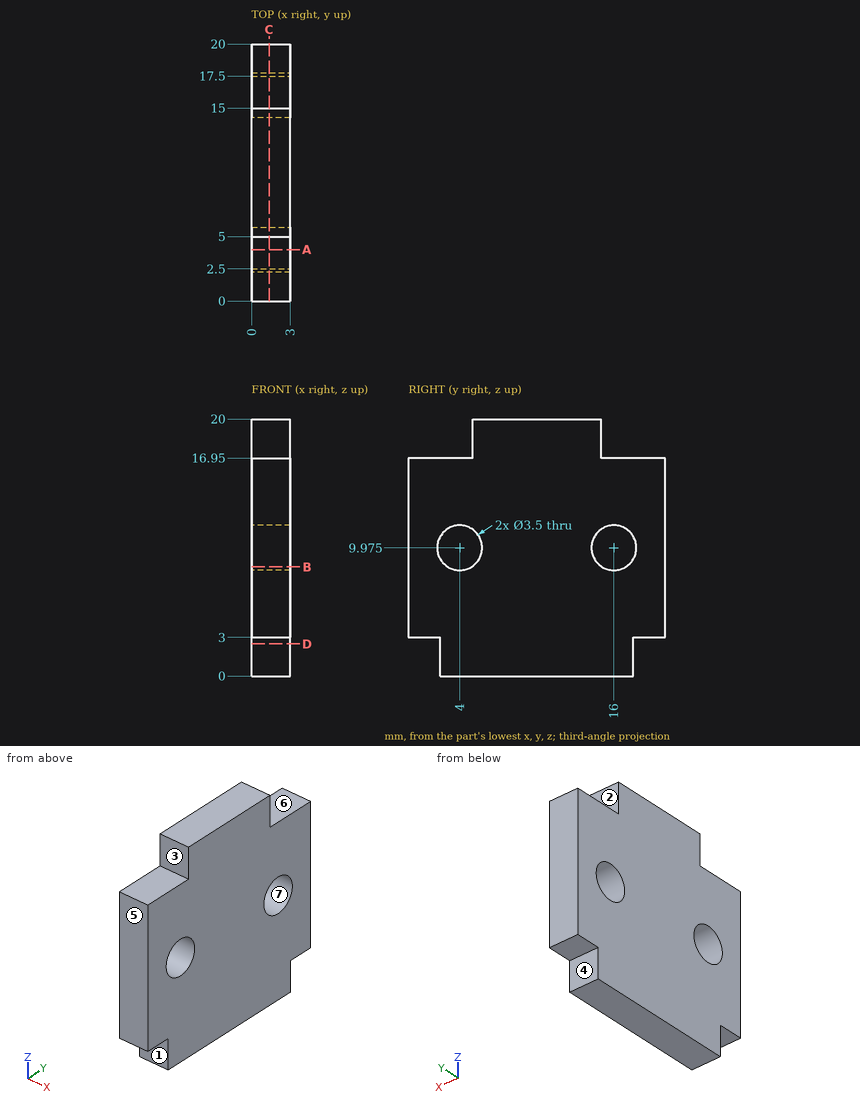
Print and shaded views of the part. All mm, measured from the part's lowest x, y and z. A direction names the side the tool comes from. Give positions to 0.01 mm unless a question says otherwise; leave off trailing zeros. Loops run counter-clockwise (first coordinate to the right, second up) from the corner with the lowest first, then second, coordinate; pieces in that order, holes last.
1) Flat gauge pins, fed straight in: pin 1 Ø0.9 at (x, y) = (1, 2.5) entering from +Z; pin 2 Ø0.9 at (x, z) = (1.5, 2) entering from -Y; pin 3 Ø3 at (y, z) = (4, 9.975) entering from -X; pin 4 Ø1.2 at (x, y) = (1, 1) entering from -Z. Where does each tip first touch, or does it go through?
2) Tool access for the marked faces 1, 2, 3 and 4: list every direction of +Z, -Z, +X, -X, +Y, -Y with a clear straight run to the whole face (end or side of a thin tool).
3) Saw through at D-D (z = 2.5). Write the cut outline in (x, y).
4) Saw through at C-C (x = 1.35). Write the cut outline in (y, z) (3 decimals).
5) Wall check: line 1 (Z direction, x = 0.65, y = 16) (3 decimals); line 2 (Y direction, x = 0.9, z = 11.5); line 3 (Y direction, x = 0.65, z = 2.5). Give the ranges that are in metal, low to high.
6) Saw through at A-A (y = 4). Write the cut outline in (x, z) (3 decimals), plus the area to 4 significant figures.
7) Saw through at B-B (z = 8.5). Write the cut outline in (x, y).
8) Pull direction Z, two halves, no side cores. Call the marked faces 5, 6 and 7: +Z half, -Z half, draft (parallel to the pull), parting line (faces both ways), or undercut.
Answer block:
1. pin 1: stops at z = 16.95
1. pin 2: stops at y = 2.5
1. pin 3: passes through
1. pin 4: stops at z = 3
2. face 1: -Z, +X, -X, -Y
2. face 2: +Z, +X, -X, +Y
2. face 3: +Z, +X, -X, -Y
2. face 4: -Z, +X, -X, +Y
3. outline: (0, 2.5) - (3, 2.5) - (3, 17.5) - (0, 17.5) - close
4. outline: (0, 3) - (2.5, 3) - (2.5, 0) - (17.5, 0) - (17.5, 3) - (20, 3) - (20, 16.95) - (15, 16.95) - (15, 20) - (5, 20) - (5, 16.95) - (0, 16.95) - close; hole circle Ø3.5 at (4, 9.975); hole circle Ø3.5 at (16, 9.975)
5. line 1: z = 0 to 8.225, 11.725 to 16.95
5. line 2: y = 0 to 3.14, 4.86 to 15.14, 16.86 to 20
5. line 3: y = 2.5 to 17.5
6. outline: (0, 0) - (3, 0) - (3, 8.225) - (0, 8.225) - close; (0, 11.725) - (3, 11.725) - (3, 16.95) - (0, 16.95) - close
6. area: 40.35 mm2
7. outline: (0, 0) - (3, 0) - (3, 3.06) - (0, 3.06) - close; (0, 4.94) - (3, 4.94) - (3, 15.06) - (0, 15.06) - close; (0, 16.94) - (3, 16.94) - (3, 20) - (0, 20) - close
8. face 5: draft
8. face 6: +Z half
8. face 7: undercut
